from build123d import *

# Parameters (mm, degrees)
SKETCH1_R                = 35
BOSS_EXTRUDE1_DEPTH      = 800
SKETCH2_R                = 75
BOSS_EXTRUDE2_DEPTH      = 5
FILLET1_R                = 10
F_8_0_8_DIAMETER_HOLE1_D = 8
CIRPATTERN1_COUNT        = 5


with BuildPart() as part:
    # Sketch1 → Boss-Extrude1 (new body)
    with BuildSketch(Plane(origin=(0, 0, 0), x_dir=(1, 0, 0), z_dir=(0, 1, 0))):
        with Locations(Location((0, 0, 0), (0, 0, 270))):
            Circle(SKETCH1_R)
    extrude(amount=BOSS_EXTRUDE1_DEPTH)

    # Sketch2 → Boss-Extrude2 (add)
    with BuildSketch(Plane(origin=(0, 800, 0), x_dir=(1, 0, 0), z_dir=(0, 1, 0))):
        with Locations(Location((0, 0, 0), (0, 0, 270))):
            Circle(SKETCH2_R)
    extrude(amount=BOSS_EXTRUDE2_DEPTH)

    # Fillet1
    fillet1_edges = [part.edges().sort_by_distance(p)[0] for p in [
        (0, 800, -35),
    ]]
    fillet(fillet1_edges, radius=FILLET1_R)

    # Ø8.0 (8) Diameter Hole1 (through all)
    with Locations(Plane(origin=(0, 805, 0), x_dir=(1, 0, 0), z_dir=(0, 1, 0))):
        with Locations((0, -57.858005833)):
            f_8_0_8_diameter_hole1 = Hole(F_8_0_8_DIAMETER_HOLE1_D / 2)

    # CirPattern1: Ø8.0 (8) Diameter Hole1 ×5 about axis
    cirpattern1_axis = Axis((0, 0, 0), (0, 1, 0))
    for i in range(1, CIRPATTERN1_COUNT):
        add(f_8_0_8_diameter_hole1.rotate(cirpattern1_axis, i * 360 / CIRPATTERN1_COUNT), mode=Mode.SUBTRACT)


solid = part.part
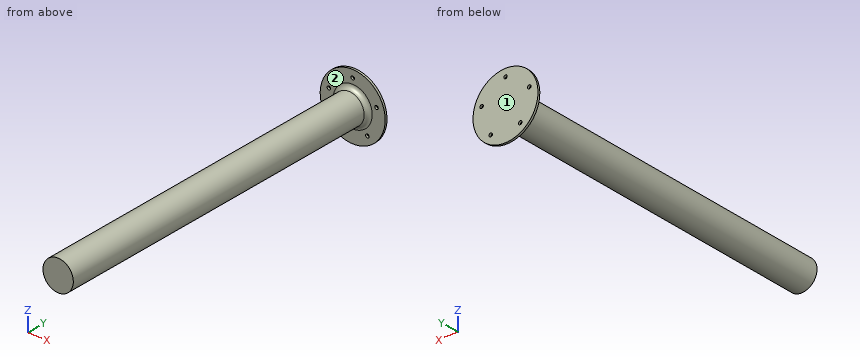
Build history of the part. All positions in model axes, mm. Face numbers are marked on the shaded views. A direction names the side the tool comes from. Round coordinates to 2 decimals unless told otherwise and drop trailing zeros. Loops run counter-clockwise (first coordinate to the right, second up) from the corner with the lowest first, then second, coordinate; pieces in that order, holes last. Notation, with made-up numbers: (17.5, -23) -> (75.5, -23) arc R17 ccw to (75.5, 9) -> close; hole circle Ø1 at (34.25, -36.75). An arc over 180 degrees is marked (long way). Use CSV: the item, a comma, the result in double quotes. Start each with the question number.
Q1. Saw through at A-A on z = 0. Give the cut face in (x, y).
Q2. Flat gauge pins, fed straight in: pin 1 Ø3 at (x, y) = (23, 283) entering from -Z; pin 2 Ø9 at (x, z) = (0, 57.86) entering from -Y; pin 3 Ø8 at (x, y) = (-1, 567.5) entering from +Z. Where does each tip first touch, or does it go through?
Q3. Which spindle directions (+Z, -Z, +X, -X, +Y, -Y) get a long thin tool onto all of the face, cutting with end or side? Do the marked faces 1 and 2. Say none if no direction does.
Q4. Saw through at B-B on y = 597.5. Give the cut face in (x, z).
Q5. Drill centre lines: L1, parallel to Y at x = -40.5, z = 46; L2, parallel to Z at x = 9, y = 637.5; L3, parallel to Y at x = 36, z = 16. Where is each one in solid material? Low to high.
Solutions:
1,outline,"(-75, 800) -> (-45, 800) arc R10 cw to (-35, 790) -> (-35, 0) -> (35, 0) -> (35, 790) arc R10 cw to (45, 800) -> (75, 800) -> (75, 805) -> (-75, 805) -> close"
2,pin 1,"stops at z = -27.62"
2,pin 2,"stops at y = 800"
2,pin 3,"stops at z = 35"
3,face 1,"+Z, -Z, +X, -X, +Y"
3,face 2,"-Y"
4,outline,"circle Ø70 at (0, 0)"
5,L1,"y = 800 to 805"
5,L2,"z = -33.82 to 33.82"
5,L3,"y = 798.28 to 805"
